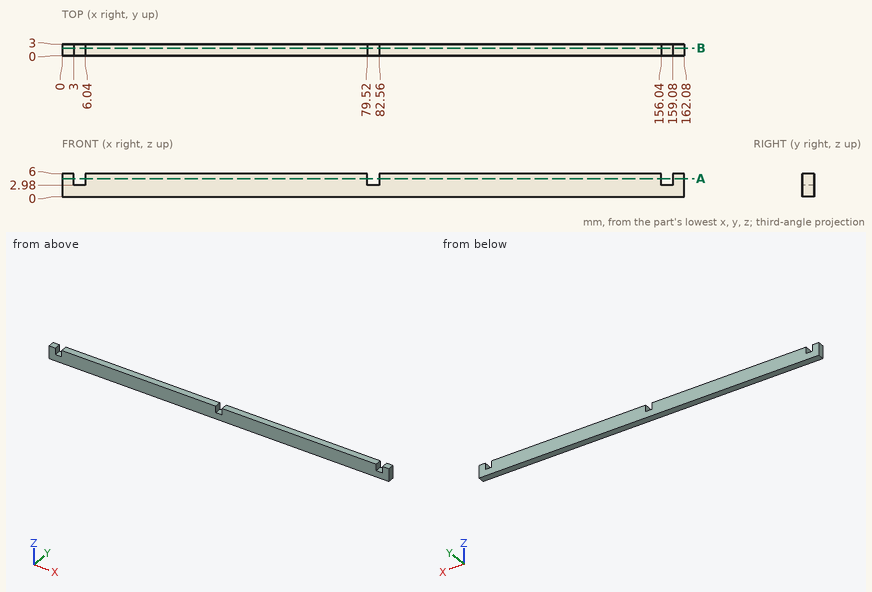
Verification items for this drawing (mm, ordinates from the low corner). Give positions to 0.01 mm unless a question says otherwise; leave off trailing zeros. Loops run counter-clockwise (first coordinate to the right, second up) from the corner with the lowest first, then second, coordinate; pieces in that order, holes last. Notation, with made-up numbers: (-28, 10) - (-19, 10) arc R21 ccw to (-19, 48) - close; hole circle Ø1 at (38, 7). An arc over 180 degrees is marked (long way). Write item = value, one per line. Start each with the question number.
Q1. Depth check by flat-ended pin: P1, Ø1.5, axis at x = 4.5, y = 2, coming from the +Z side; P2, Ø1.5, axis at y = 1.5, z = 4, coming from the -X side. Enter the tip coordinate at first touch or a pass-through.
Q2. Cross-section at A-A, the plane z = 4.7. Enter the section's corners in (x, y).
Q3. Thickness scan on line 1 (X direction, y = 0.9, z = 4.6). Record the ranges inside material, lowest first.
Q4. Cross-section at B-B, the plane y = 1.9. Enter the section's corners in (x, z).
Answer key:
q1.P1 = 2.98
q1.P2 = 0
q2.outline = (0, 0) - (3, 0) - (3, 3) - (0, 3) - close; (6.04, 0) - (79.52, 0) - (79.52, 3) - (6.04, 3) - close; (82.56, 0) - (156.04, 0) - (156.04, 3) - (82.56, 3) - close; (159.08, 0) - (162.08, 0) - (162.08, 3) - (159.08, 3) - close
q3.line_1 = 0 to 3, 6.04 to 79.52, 82.56 to 156.04, 159.08 to 162.08
q4.outline = (0, 0) - (162.08, 0) - (162.08, 6) - (159.08, 6) - (159.08, 2.98) - (156.04, 2.98) - (156.04, 6) - (82.56, 6) - (82.56, 2.98) - (79.52, 2.98) - (79.52, 6) - (6.04, 6) - (6.04, 2.98) - (3, 2.98) - (3, 6) - (0, 6) - close
